from build123d import *

# Parameters (mm, degrees)
BOSS_EXTRUDE1_DEPTH = 20
BOSS_EXTRUDE2_DEPTH = 5
BOSS_EXTRUDE4_DEPTH = 5
SKETCH8_R           = 3.175
CUT_EXTRUDE2_DEPTH  = 47.2699694
SKETCH9_R           = 6
CUT_EXTRUDE3_DEPTH  = 5
SKETCH10_R          = 3.175
CUT_EXTRUDE4_DEPTH  = 47.269969478
SKETCH11_R          = 6
CUT_EXTRUDE5_DEPTH  = 5


with BuildPart() as part:
    # Sketch1 → Boss-Extrude1 (new body)
    with BuildSketch(Plane.XY):
        with BuildLine():
            Line((16.65, 0), (23.618063018, -1.228657513))
            ThreePointArc((23.618063018, -1.228657513), (0, 23.65), (-23.618063018, -1.228657513))
            Line((-23.618063018, -1.228657513), (-16.65, 0))
            ThreePointArc((-16.65, 0), (0, 16.65), (16.65, 0))
        make_face()
    extrude(amount=BOSS_EXTRUDE1_DEPTH)

    # Sketch2 → Boss-Extrude2 (add)
    with BuildSketch(Plane(origin=(0.502058932, 2.847317693, 0), x_dir=(-0.9848077530122079, 0.1736481776669312, 0), z_dir=(-0.1736481776669312, -0.9848077530122079, 0))):
        with BuildLine():
            Line((-26.397049088, 0), (-16.397049088, 0))
            Line((-16.397049088, 0), (-16.397049088, -20))
            Line((-16.397049088, -20), (-26.397049088, -20))
            ThreePointArc((-26.397049088, -20), (-36.397049088, -10), (-26.397049088, 0))
        make_face()
    extrude(amount=-BOSS_EXTRUDE2_DEPTH)

    # Sketch6 → Boss-Extrude4 (add)
    with BuildSketch(Plane(origin=(-0.502058932, 2.847317693, 0), x_dir=(0.9848077530122087, 0.173648177666927, 0), z_dir=(0.173648177666927, -0.9848077530122087, 0))):
        with BuildLine():
            Line((-26.397049088, 20), (-16.397049088, 20))
            Line((-16.397049088, 20), (-16.397049088, 0))
            Line((-16.397049088, 0), (-26.397049088, 0))
            ThreePointArc((-26.397049088, 0), (-36.397049088, 10), (-26.397049088, 20))
        make_face()
    extrude(amount=-BOSS_EXTRUDE4_DEPTH)

    # Sketch8 → Cut-Extrude2 (cut, through all)
    with BuildSketch(Plane(origin=(-1.37029982, 7.771356458, 0), x_dir=(0.9848077530122087, 0.173648177666927, 0), z_dir=(-0.173648177666927, 0.9848077530122087, 0))):
        with Locations(Location((-26.397049088, -10, 0), (0, 0, 180))):
            Circle(SKETCH8_R)
    extrude(amount=-CUT_EXTRUDE2_DEPTH, mode=Mode.SUBTRACT)

    # Sketch9 → Cut-Extrude3 (cut)
    with BuildSketch(Plane(origin=(-1.37029982, 7.771356458, 0), x_dir=(0.9848077530122087, 0.173648177666927, 0), z_dir=(-0.173648177666927, 0.9848077530122087, 0))):
        with Locations((-26.397049088, -10)):
            Circle(SKETCH9_R)
    extrude(amount=CUT_EXTRUDE3_DEPTH, mode=Mode.SUBTRACT)

    # Sketch10 → Cut-Extrude4 (cut, through all)
    with BuildSketch(Plane(origin=(1.37029982, 7.771356458, 0), x_dir=(0.9848077530122079, -0.1736481776669312, 0), z_dir=(0.1736481776669312, 0.9848077530122079, 0))):
        with Locations(Location((26.397049088, -10, 0), (0, 0, 180))):
            Circle(SKETCH10_R)
    extrude(amount=-CUT_EXTRUDE4_DEPTH, mode=Mode.SUBTRACT)

    # Sketch11 → Cut-Extrude5 (cut)
    with BuildSketch(Plane(origin=(1.37029982, 7.771356458, 0), x_dir=(0.9848077530122079, -0.1736481776669312, 0), z_dir=(0.1736481776669312, 0.9848077530122079, 0))):
        with Locations((26.397049088, -10)):
            Circle(SKETCH11_R)
    extrude(amount=CUT_EXTRUDE5_DEPTH, mode=Mode.SUBTRACT)


solid = part.part
Source: CAD feature listing. Evaluate the final solid. Frame: model axes, mm. A direction names the side the tool comes from. Coordinates: 2 decimals unless noted, no trailing zeros. Loops run counter-clockwise (first coordinate to the right, second up) from the corner with the lowest first, then second, coordinate; pieces in that order, holes last. Notation, with made-up numbers: (48.5, 72) -> (105.5, 72) arc R35 cw to (105.5, 105) -> close; hole circle Ø8 at (4.25, 27). An arc over 180 degrees is marked (long way). Answer in a Markdown table with one row per item. Add a question column.
Q1. Section C-C on z = 18.5. Return the cut outline in (x, y), and give its area (3 significant figures).
Q2. Reachability of faces 4 (the face through (0.465, 23.645, 9.86)), 5 (the face through (-21.728, 5.764, 10.069)) from +Z, -Z, +X, -X, +Y, -Y: full face, straight path, thin tool, end or side. Return the list, or none.
Q3. Section D-D on y = 20.25. Return the cut outline in (x, z).
Q4. Ray query, line 1 along X through (y, z) = (0.5, 1.5); line 2 along X through (y, z) = (8, 10.75); line 3 along Y through (x, z) = (-21.5, 17.25). Return the intervals inside material, ascending.
Q5. Contact query for flat-ended pins moving along their axis: pin 1 Ø4 at (y, z) = (1.5, 7.5) entering from -X; pin 2 Ø8 at (x, z) = (10.5, 2.5) entering from +Y; pin 3 Ø12 at (x, y) = (9.5, -0.5) entering from -Z; pin 4 Ø2 at (x, z) = (2.5, 3.5) entering from +Y. Output: stop coordinate, or through.
Q6. Pull-direction query (Z, two-part tool) for faces 1 (the face through (0, 18, 0)), 2 (the face through (21.728, 5.763, 9.931)), 3 (the face through (-36.772, -1.045, 9.78)); classes: pulls with the +Z half, pulls with the -Z half, needs draft (parallel to the pull), parting line crosses it, or undercut.
Q7. Section B-B on x = 0. Return the cut outline in (y, z).
Q8. Section A-A on z = 7.75. Return the cut outline in (x, y).
Computed values:
| question | item | result |
|---|---|---|
| 1 | outline | (-32.55, 2.27) -> (-31.69, -2.65) -> (-16.65, 0) arc R16.65 cw to (16.65, 0) -> (31.69, -2.65) -> (32.55, 2.27) -> (23.33, 3.9) arc R23.65 ccw to (-23.33, 3.9) -> close |
| 1 | area | 539 mm^2 |
| 2 | face 4 | +Z, -Z, +Y |
| 2 | face 5 | -X |
| 3 | outline | (-12.22, 0) -> (12.22, 0) -> (12.22, 20) -> (-12.22, 20) -> close |
| 4 | line 1 | x = -32.24 to -16.64, 16.64 to 32.24 |
| 4 | line 2 | x = -22.17 to -14.6, 14.6 to 22.17 |
| 4 | line 3 | y = -0.86 to 9.85 |
| 5 | pin 1 | stops at x = -37.2 |
| 5 | pin 2 | stops at y = 22.74 |
| 5 | pin 3 | passes through |
| 5 | pin 4 | stops at y = 23.6 |
| 6 | face 1 | pulls with the -Z half |
| 6 | face 2 | undercut |
| 6 | face 3 | parting line crosses it |
| 7 | outline | (16.65, 0) -> (23.65, 0) -> (23.65, 20) -> (16.65, 20) -> close |
| 8 | outline | (-36.96, 1.5) -> (-36.09, -3.43) -> (-28.7, -2.13) -> (-29.57, 2.8) -> close; (-25.16, 3.58) -> (-24.29, -1.35) -> (-16.65, 0) arc R16.65 cw to (16.65, 0) -> (24.29, -1.35) -> (25.16, 3.58) -> (21.89, 4.15) -> (22.46, 7.4) arc R23.65 ccw to (-22.46, 7.4) -> (-21.89, 4.15) -> close; (28.7, -2.13) -> (36.09, -3.43) -> (36.96, 1.5) -> (29.57, 2.8) -> close |
